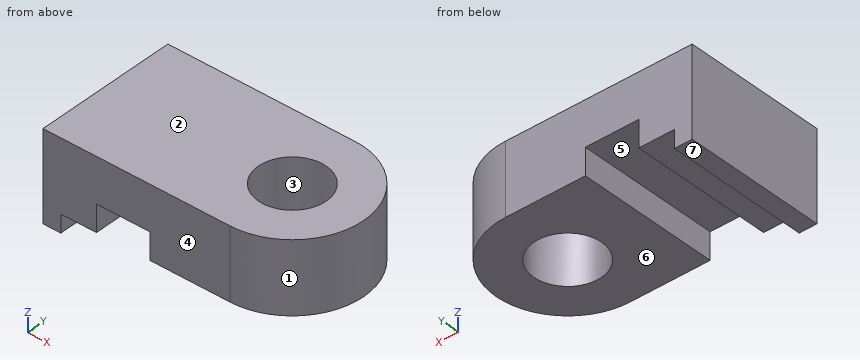
from build123d import *

# Parameters (mm, degrees)
SKETCH_1_R          = 1.9
EXTRUDE_1_DEPTH     = 4
SKETCH_2_W          = 3
SKETCH_2_H          = 1.5
CUT_EXTRUDE_1_DEPTH = 14.793114224
SKETCH_3_W          = 1
SKETCH_3_H          = 8
EXTRUDE_2_DEPTH     = 1


with BuildPart() as part:
    # 草图1 → 凸台-拉伸1 (new body)
    with BuildSketch(Plane.XY):
        with BuildLine():
            Line((0, 4), (-10.5, 4))
            Line((-10.5, 4), (-10.5, -4))
            Line((-10.5, -4), (0, -4))
            ThreePointArc((0, -4), (4, 0), (0, 4))
        make_face()
        Circle(SKETCH_1_R, mode=Mode.SUBTRACT)
    extrude(amount=EXTRUDE_1_DEPTH)

    # 草图2 → 切除-拉伸1 (cut, through all)
    with BuildSketch(Plane(origin=(0, 4, 0), x_dir=(1, 0, 0), z_dir=(0, 1, 0))):
        with Locations((-6, -0.75)):
            Rectangle(SKETCH_2_W, SKETCH_2_H)
    extrude(amount=-CUT_EXTRUDE_1_DEPTH, mode=Mode.SUBTRACT)

    # 草图3 → 凸台-拉伸2 (add)
    with BuildSketch(Plane(origin=(0, 0, 0), x_dir=(-1, 0, 0), z_dir=(0, 0, -1))):
        with Locations((10, 0)):
            Rectangle(SKETCH_3_W, SKETCH_3_H)
    extrude(amount=EXTRUDE_2_DEPTH)


solid = part.part
CAD build for the part. Positions are in the model's coordinates, mm. Face numbers are marked on the shaded views. A direction names the side the tool comes from. Give positions to 0.01 mm unless a question says otherwise; leave off trailing zeros. Write each loop counter-clockwise with the first axis right and the second up, starting at its lowest first coordinate (ties: lowest second). Pieces come first, ordered by that corner, then holes. Notation, with made-up numbers: M -6,9 L 15,9 A18 cw 15,19 Z; hole C 56,-26 d1. An arc over 180 degrees is marked long. Put each result on its own line as item: value. Start each with the question number.
(1) Band-saw the part on C-C, the plane z = 1.9. Write the cut outline in (x, y), and give its area (3 significant figures).
(2) Flat gauge pins, fed straight in: pin 1 Ø3.5 at (x, y) = (-6, 0.5) entering from -Z; pin 2 Ø1.5 at (x, y) = (-6, -1.5) entering from -Z; pin 3 Ø0.5 at (y, z) = (1.5, -0.5) entering from +X. Where does each tip first touch, or does it go through?
(3) Mould opens along Y. For the marked faces 1, 2, 3 and 4 say: +Y half, -Y half, draft (parallel to the pull), parting line (faces both ways), or undercut.
(4) Which spindle directions (+Z, -Z, +X, -X, +Y, -Y) get a long thin tool onto all of the face, cutting with end or side? Do the marked faces 5, 6 and 7. Say none if no direction does.
(5) Band-saw the part on D-D, the plane x = 1.75. Write the cut outline in (y, z).
(6) Band-saw the part on A-A, the plane z = 0.5. Write the cut outline in (x, y).
(7) Band-saw the part on B-B, the plane y = 0. Write the cut outline in (x, z).
(8) Probe L1, parallel to Z at x = -5.5, y = 1.75; L2, parallel to Z at x = 2.5, y = -2.25; L3, parallel to X at y = -2.25, z = -0.4. List the from-to ranges inside material, lowest first.
Response values:
1. outline: M -10.5,-4 L 0,-4 A4 ccw 0,4 L -10.5,4 Z; hole C 0,0 d3.8
1. area: 97.8 mm2
2. pin 1: stops at z = 0
2. pin 2: stops at z = 1.5
2. pin 3: stops at x = -9.5
3. face 1: parting line
3. face 2: draft
3. face 3: undercut
3. face 4: -Y half
4. face 5: -Z, +Y, -Y
4. face 6: -Z, +X, +Y, -Y
4. face 7: -Z, +X, -X, +Y, -Y
5. outline: M -3.6,0 L -0.74,0 L -0.74,4 L -3.6,4 Z; M 0.74,0 L 3.6,0 L 3.6,4 L 0.74,4 Z
6. outline: M -10.5,-4 L -7.5,-4 L -7.5,4 L -10.5,4 Z; M -4.5,-4 L 0,-4 A4 ccw 0,4 L -4.5,4 Z; hole C 0,0 d3.8
7. outline: M -10.5,-1 L -9.5,-1 L -9.5,0 L -7.5,0 L -7.5,1.5 L -4.5,1.5 L -4.5,0 L -1.9,0 L -1.9,4 L -10.5,4 Z; M 1.9,0 L 4,0 L 4,4 L 1.9,4 Z
8. L1: z = 1.5 to 4
8. L2: z = 0 to 4
8. L3: x = -10.5 to -9.5
